Print and shaded views of the part. All mm, measured from the part's lowest x, y and z. A direction names the side the tool comes from. Give positions to 0.01 mm unless a question says otherwise; leave off trailing zeros. Write each loop counter-clockwise with the first axis right and the second up, starting at its lowest first coordinate (ties: lowest second). Pieces come first, ordered by that corner, then holes. Notation, with made-up numbers: (53.5, 16) -> (104.5, 16) arc R16 cw to (104.5, 25) -> close; hole circle Ø3 at (37.5, -1.75). An arc over 180 degrees is marked (long way). Put each result on its own line as item: value.
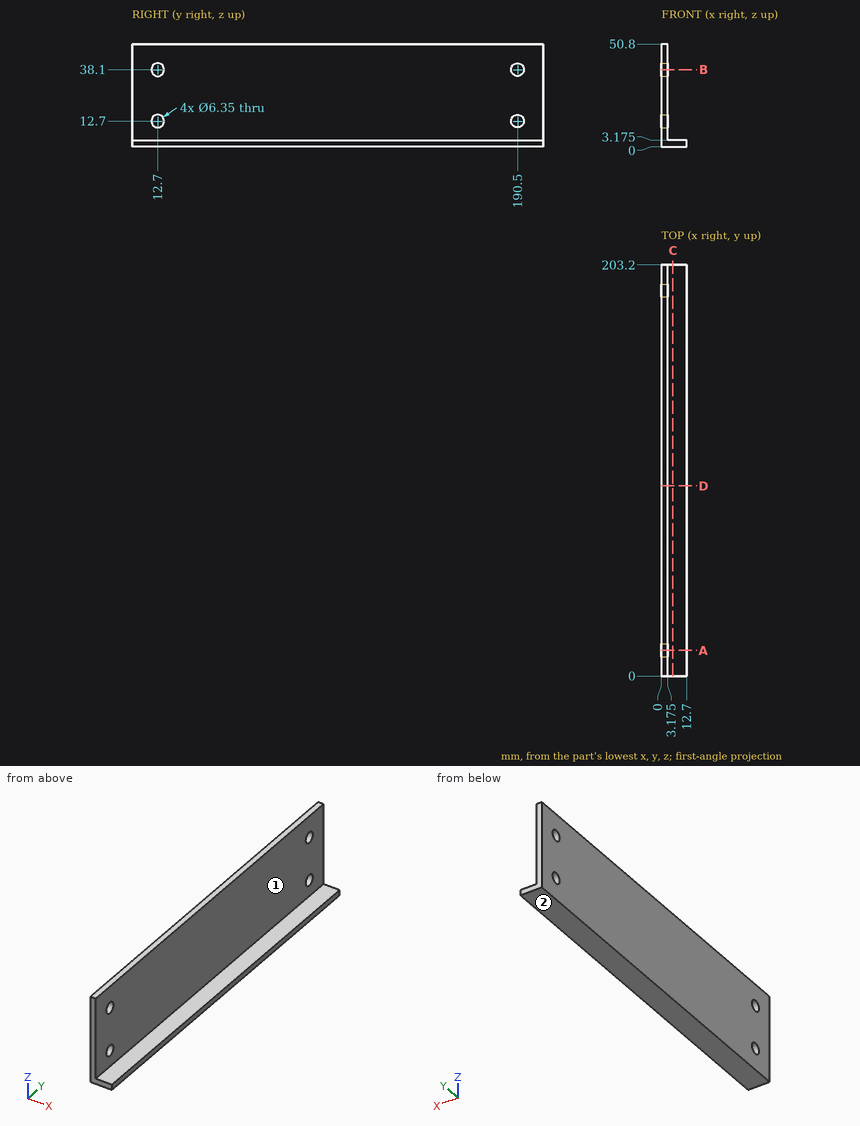
1) Pin check, flat tips, straight feed: pin 1 (3 mm diameter, centred on x = 6.5, y = 94.5, fed in from +Z) (3 decimals); pin 2 (4 mm diameter, centred on y = 12.7, z = 12.7, fed in from -X); pin 3 (8.5 mm diameter, centred on y = 190.5, z = 12.7, fed in from +X) (3 decimals). Stop position of each tip, or through.
Filled sheet:
pin 1: z = 3.175
pin 2: through
pin 3: x = 3.175
2) Slice it at B-B (z = 38.1). Write the cut outline in (x, y) (3 decimals), plus the area to 3 significant figures.
Filled sheet:
outline: (0, 0) -> (3.175, 0) -> (3.175, 9.525) -> (0, 9.525) -> close; (0, 15.875) -> (3.175, 15.875) -> (3.175, 187.325) -> (0, 187.325) -> close; (0, 193.675) -> (3.175, 193.675) -> (3.175, 203.2) -> (0, 203.2) -> close
area: 605 mm2
3) Wall check: L1, parallel to Z at x = 1.4, y = 12.7 (3 decimals); L2, parallel to Y at x = 1.25, z = 37.5; L3, parallel to Z at x = 5.5, y = 179.5 (3 decimals). Give the ranges that are in metal, low to high.
Filled sheet:
L1: 0 to 9.525, 15.875 to 34.925, 41.275 to 50.8
L2: 0 to 9.58, 15.82 to 187.38, 193.62 to 203.2
L3: 0 to 3.175
4) Slice it at A-A (y = 12.7). Write the cut outline in (x, z) (3 decimals), plus the area to 3 significant figures.
Filled sheet:
outline: (0, 0) -> (12.7, 0) -> (12.7, 3.175) -> (3.175, 3.175) -> (3.175, 9.525) -> (0, 9.525) -> close; (0, 15.875) -> (3.175, 15.875) -> (3.175, 34.925) -> (0, 34.925) -> close; (0, 41.275) -> (3.175, 41.275) -> (3.175, 50.8) -> (0, 50.8) -> close
area: 151 mm2
5) Tool access for the marked faces 1 and 2: list every direction of +Z, -Z, +X, -X, +Y, -Y with a clear straight run to the whole face (end or side of a thin tool).
Filled sheet:
face 1: +Z, +X, +Y, -Y
face 2: -Z, +X, -X, +Y, -Y
6) Slice it at D-D (y = 94). Write the cut outline in (x, z) (3 decimals), plus the area to 3 significant figures.
Filled sheet:
outline: (0, 0) -> (12.7, 0) -> (12.7, 3.175) -> (3.175, 3.175) -> (3.175, 50.8) -> (0, 50.8) -> close
area: 192 mm2
7) Slice it at C-C (x = 5.75). Write the cut outline in (y, z) (3 decimals), plus the area to 3 significant figures.
Filled sheet:
outline: (0, 0) -> (203.2, 0) -> (203.2, 3.175) -> (0, 3.175) -> close
area: 645 mm2
